```python
from build123d import *

# Parameters (mm, degrees)
SKETCH_1_W          = 11.2
SKETCH_1_H          = 9.2
EXTRUDE_1_DEPTH     = 60
SKETCH_1_12_W       = 5.2
SKETCH_1_12_H       = 3.2
CUT_EXTRUDE_1_DEPTH = 18
SKETCH_2_R          = 9.5
CUT_EXTRUDE_2_DEPTH = 61.959002617
FILLET_1_R          = 2
SKETCH_3_R          = 40
EXTRUDE_2_DEPTH     = 4
EXTRUDE_3_DEPTH     = 1.5
EXTRUDE_4_DEPTH     = 1.5
FILLET_2_R          = 10


with BuildPart() as part:
    # Sketch 1 → Extrude 1 (new body)
    with BuildSketch(Plane(origin=(0, 0, 0), x_dir=(1, 0, 0), z_dir=(0, 1, 0))):
        Rectangle(SKETCH_1_W, SKETCH_1_H)
    extrude(amount=EXTRUDE_1_DEPTH)

    # Sketch 1_12 → Cut-Extrude 1 (cut)
    with BuildSketch(Plane(origin=(0, 0, 0), x_dir=(1, 0, 0), z_dir=(0, 1, 0))):
        Rectangle(SKETCH_1_12_W, SKETCH_1_12_H)
    extrude(amount=CUT_EXTRUDE_1_DEPTH, mode=Mode.SUBTRACT)

    # Sketch 2 → Cut-Extrude 2 (cut, through all)
    with BuildSketch(Plane(origin=(0, 0, -4.6), x_dir=(-1, 0, 0), z_dir=(0, 0, -1))):
        with Locations((0, -7)):
            Circle(SKETCH_2_R)
    extrude(amount=-CUT_EXTRUDE_2_DEPTH, mode=Mode.SUBTRACT)

    # Fillet 1
    fillet_1_edges = [part.edges().sort_by_distance(p)[0] for p in [
        (-2.6, 2.137286249, 0),
        (0, 2.5, -1.6),
        (0, 2.5, 1.6),
        (2.6, 2.137286249, 0),
    ]]
    fillet(fillet_1_edges, radius=FILLET_1_R)

    # Sketch 3 → Extrude 2 (add)
    with BuildSketch(Plane(origin=(0, 60, 0), x_dir=(1, 0, 0), z_dir=(0, 1, 0))):
        with Locations(Location((0, 0, 0), (0, 0, 270))):
            Circle(SKETCH_3_R)
    extrude(amount=EXTRUDE_2_DEPTH)

    # Sketch 4 → Extrude 3 (add, symmetric)
    with BuildSketch(Plane.ZY):
        with BuildLine():
            ThreePointArc((-20.1, 60), (-19.591568767, 58.488823688), (-18.273076923, 57.592310764))
            Line((-18.273076923, 57.592310764), (-9.847432928, 55.236896099))
            Line((-9.847432928, 55.236896099), (-7.061421083, 39.5625))
            ThreePointArc((-7.061421083, 39.5625), (-6.205654072, 38.083786285), (-4.6, 37.5))
            Line((-4.6, 37.5), (-4.6, 60))
            Line((-4.6, 60), (-20.1, 60))
        make_face()
    extrude_3 = extrude(amount=EXTRUDE_3_DEPTH, both=True)

    # Sketch 5 → Extrude 4 (add, symmetric)
    with BuildSketch(Plane.XY):
        with BuildLine():
            ThreePointArc((-23.6, 60), (-23.057203403, 58.444572458), (-21.664516129, 57.564569537))
            Line((-21.664516129, 57.564569537), (-10.81412887, 55.04952396))
            Line((-10.81412887, 55.04952396), (-8.061421083, 39.5625))
            ThreePointArc((-8.061421083, 39.5625), (-7.205654072, 38.083786285), (-5.6, 37.5))
            Line((-5.6, 37.5), (-5.6, 60))
            Line((-5.6, 60), (-23.6, 60))
        make_face()
    extrude_4 = extrude(amount=EXTRUDE_4_DEPTH, both=True)

    # Mirror 2: Extrude 3 across plane
    add(extrude_3.mirror(Plane.XY))

    # Mirror 3: Extrude 4 across plane
    add(extrude_4.mirror(Plane(origin=(0, 0, 0), x_dir=(0, 0, 1), z_dir=(1, 0, 0))))

    # Fillet 2
    fillet_2_edges = [part.edges().sort_by_distance(p)[0] for p in [
        (-10.81412887, 55.04952396, 0),
        (0, 55.236896099, 9.847432928),
        (10.81412887, 55.04952396, 0),
        (0, 55.236896099, -9.847432928),
    ]]
    fillet(fillet_2_edges, radius=FILLET_2_R)


solid = part.part
```
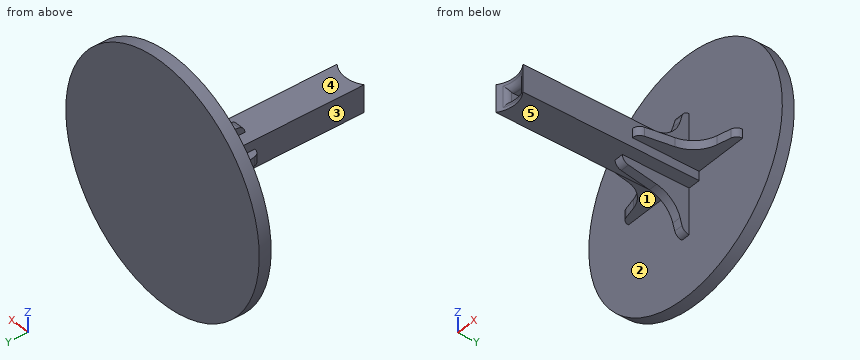
Input: part model. Units: mm. Frame: model coordinates. Face numbers are marked on the shaded views. A direction names the side the tool comes from. Round coordinates to 2 decimals unless told otherwise and drop trailing zeros. Loops run counter-clockwise (first coordinate to the right, second up) from the corner with the lowest first, then second, coordinate; pieces in that order, holes last. Notation, with made-up numbers: M -3,12.25 L 12,12.25 A28 cw 12,38.25 Z; hole C 8,57 d2. An arc over 180 degrees is marked long. Answer in a Markdown table with one row per item. Add a question column.
1. Section B-B (z = 0). Output: boundary loops of the cut face in (x, y).
2. Set-up query: the marked faces 1, 2, 3, 4 and 5. Return all of +Z, -Z, +X, -X, +Y, -Y with unobstructed straight access to the full face (end or side cutting, diameter ignored); none if empty.
3. Section C-C (y = 44.5). Output: boundary loops of the cut face in (x, z), and give its area (3 significant figures).
4. Section A-A (x = 0). Output: boundary loops of the cut face in (y, z).
5. Section D-D (x = 12). Output: boundary loops of the cut face in (y, z).
6. Ray query, probe 1 along X at (y, z) = (12, 1.5); probe 2 along Y at (x, z) = (-30, -23); probe 3 along Z at (x, y) = (15, 58.5). Return the intervals inside material, ascending.
7. Contact query for flat-ended pins moving along their axis: pin 1 (4 mm diameter, centred on x = -1, y = 11.5, fed in from +Z); pin 2 (1.7 mm diameter, centred on y = 13.5, z = -0.5, fed in from -X); pin 3 (20 mm diameter, centred on x = 10.5, y = 49, fed in from -Z). Output: stop coordinate, or through.
Values follow:
| question | item | result |
|---|---|---|
| 1 | outline | M -40,60 L -23.6,60 A2.5 ccw -21.66,57.56 L -17.25,56.54 A10 cw -9.66,48.55 L -8.06,39.56 A2.5 ccw -5.6,37.5 L -5.6,0.67 A9.5 cw -3.8,1.71 A2 ccw -2.6,3.54 L -2.6,18 L 2.6,18 L 2.6,3.54 A2 ccw 3.8,1.71 A9.5 cw 5.6,0.67 L 5.6,37.5 A2.5 ccw 8.06,39.56 L 9.66,48.55 A10 cw 17.25,56.54 L 21.66,57.56 A2.5 ccw 23.6,60 L 40,60 L 40,64 L -40,64 Z |
| 2 | face 1 | -Z, -X, -Y |
| 2 | face 2 | -Y |
| 2 | face 3 | -X, -Y |
| 2 | face 4 | +Z, -Y |
| 2 | face 5 | -Z, -Y |
| 3 | outline | M -8.94,-1.5 L -5.6,-1.5 L -5.6,-4.6 L -1.5,-4.6 L -1.5,-7.94 L 1.5,-7.94 L 1.5,-4.6 L 5.6,-4.6 L 5.6,-1.5 L 8.94,-1.5 L 8.94,1.5 L 5.6,1.5 L 5.6,4.6 L 1.5,4.6 L 1.5,7.94 L -1.5,7.94 L -1.5,4.6 L -5.6,4.6 L -5.6,1.5 L -8.94,1.5 Z |
| 3 | area | 143 mm^2 |
| 4 | outline | M 2.5,-4.6 L 37.5,-4.6 A2.5 ccw 39.56,-7.06 L 49.05,-8.75 A10 cw 56.93,-15.9 L 57.59,-18.27 A2.5 ccw 60,-20.1 L 60,-40 L 64,-40 L 64,40 L 60,40 L 60,20.1 A2.5 ccw 57.59,18.27 L 56.93,15.9 A10 cw 49.05,8.75 L 39.56,7.06 A2.5 ccw 37.5,4.6 L 2.5,4.6 L 2.5,3.6 A2 ccw 4.5,1.6 L 18,1.6 L 18,-1.6 L 4.5,-1.6 A2 ccw 2.5,-3.6 Z |
| 5 | outline | M 53.41,-1.5 L 60,-1.5 L 60,-38.16 L 64,-38.16 L 64,38.16 L 60,38.16 L 60,1.5 L 53.41,1.5 Z |
| 6 | probe 1 | -5.6 to -2.6, 2.6 to 5.6 |
| 6 | probe 2 | 60 to 64 |
| 6 | probe 3 | -1.5 to 1.5 |
| 7 | pin 1 | z = 4.6 |
| 7 | pin 2 | x = -5.6 |
| 7 | pin 3 | z = -10.64 |
